Part model, mm, in its own coordinate system. Face numbers are marked on the shaded views. Give positions to 0.01 mm unless a question says otherwise; leave off trailing zeros. Loops run counter-clockwise (first coordinate to the right, second up) from the corner with the lowest first, then second, coordinate; pieces in that order, holes last. Notation, with made-up numbers: M -34.75,47 L -4.75,47 A20 ccw -4.75,86 Z; hole C 5,34.5 d5. An arc over 180 degrees is marked long. Answer in a Markdown table with one row per item.
from build123d import *

# Parameters (mm, degrees)
MAIN_BODY_DEPTH        = 53.8
SKETCH4_W              = 35
SKETCH4_H              = 10.428932188
SKETCH4_H_2            = 14.142135624
BOSS_EXTRUDE2_DEPTH    = 2
M2X0_4_TAPPED_HOLE2_D  = 1.6
SIDE_HOLES_D           = 2.9
FILLET1_R              = 0.5
BOSS_EXTRUDE4_START    = -10
BOSS_EXTRUDE4_DEPTH    = 10
M2_5_CLEARANCE_HOLE1_D = 2.9
M2_5_CLEARANCE_HOLE2_D = 2.9


# Read off the part's stored shape, not the designer's step: Boss-Extrude4
with BuildPart() as part:
    # Sketch1 → Main Body (new, symmetric)
    with BuildSketch(Plane.XY):
        Polygon((-7.5, 2.5), (2.5, 2.5), (2.5, -7.5), align=None)
    extrude(amount=MAIN_BODY_DEPTH, both=True)

    # Sketch4 → Boss-Extrude2 (add)
    with BuildSketch(Plane(origin=(-2.5, -2.5, 0), x_dir=(0, 0, 1), z_dir=(-0.7071067811865474, -0.7071067811865477, 0))):
        with Locations((0, 12.285533906)):
            Rectangle(SKETCH4_W, SKETCH4_H)
        Rectangle(SKETCH4_W, SKETCH4_H_2)
        with Locations((0, -12.285533906)):
            Rectangle(SKETCH4_W, SKETCH4_H)
        with BuildLine():
            Line((-17.5, -17.5), (-17.5, -7.071067812))
            Line((-17.5, -7.071067812), (-26.575364532, -7.071067812))
            ThreePointArc((-26.575364532, -7.071067812), (0, -27.5), (26.575364532, -7.071067812))
            Line((26.575364532, -7.071067812), (17.5, -7.071067812))
            Line((17.5, -7.071067812), (17.5, -17.5))
            Line((17.5, -17.5), (-17.5, -17.5))
        make_face()
        with BuildLine():
            Line((-17.5, -7.071067812), (-17.5, 7.071067812))
            Line((-17.5, 7.071067812), (-26.575364532, 7.071067812))
            ThreePointArc((-26.575364532, 7.071067812), (-27.5, 0), (-26.575364532, -7.071067812))
            Line((-26.575364532, -7.071067812), (-17.5, -7.071067812))
        make_face()
        with BuildLine():
            Line((-17.5, 7.071067812), (-17.5, 17.5))
            Line((-17.5, 17.5), (17.5, 17.5))
            Line((17.5, 17.5), (17.5, 7.071067812))
            Line((17.5, 7.071067812), (26.575364532, 7.071067812))
            ThreePointArc((26.575364532, 7.071067812), (0, 27.5), (-26.575364532, 7.071067812))
            Line((-26.575364532, 7.071067812), (-17.5, 7.071067812))
        make_face()
        with BuildLine():
            Line((26.575364532, 7.071067812), (17.5, 7.071067812))
            Line((17.5, 7.071067812), (17.5, -7.071067812))
            Line((17.5, -7.071067812), (26.575364532, -7.071067812))
            ThreePointArc((26.575364532, -7.071067812), (27.267861345, -3.565632859), (27.5, 0))
            ThreePointArc((27.5, 0), (27.267861345, 3.565632859), (26.575364532, 7.071067812))
        make_face()
    extrude(amount=-BOSS_EXTRUDE2_DEPTH)

    # M2x0.4 Tapped Hole2 (through all)
    with Locations(Plane(origin=(-2.5, -2.5, 0), x_dir=(-0.7071067811865477, 0.7071067811865474, 0), z_dir=(-0.7071067811865474, -0.7071067811865477, 0))):
        with Locations((-21, 0), (14, 21), (14, -21)):
            Hole(M2X0_4_TAPPED_HOLE2_D / 2)

    # Side holes (through all)
    with Locations(Plane.XY.offset(53.8)):
        with Locations((-1, -1)):
            Hole(SIDE_HOLES_D / 2)

    # Sketch8 → Revolve1 (revolve)
    with BuildSketch(Plane(origin=(0, 0, 0), x_dir=(0, 0, 1), z_dir=(0.7071067811865476, -0.7071067811865476, 0)), mode=Mode.PRIVATE) as revolve1_sk:
        with BuildLine():
            Line((0, 3.535533906), (0, 4.535533906))
            ThreePointArc((0, 4.535533906), (-4.596194078, 6.439339828), (-6.5, 11.035533906))
            Line((-6.5, 11.035533906), (-12, 3.535533906))
            Line((-12, 3.535533906), (0, 3.535533906))
        make_face()
    revolve(revolve1_sk.sketch.rotate(Axis((-2.5, -2.5, 0), (-0.7071067811865476, -0.7071067811865476, 0)), 270), axis=Axis((-2.5, -2.5, 0), (-0.7071067811865476, -0.7071067811865476, 0)))

    # Fillet1
    fillet1_edges = [part.edges().sort_by_distance(p)[0] for p in [
        (-3.207106781, -12.399494937, 0),
    ]]
    fillet(fillet1_edges, radius=FILLET1_R)

    # Boss-Extrude4 outline → Boss-Extrude4 (add)
    with BuildSketch(Plane(origin=(2.5, 0, 0), x_dir=(0, 0, -1), z_dir=(1, 0, 0)).offset(BOSS_EXTRUDE4_START)):
        Polygon((53.8, 33.99997125), (-53.8, 33.99997125), (-53.8, 23.99997125), (-14.986093738, 13.249985625), (-53.8, 2.5), (-23.827812525, 2.5), (0, 9.099403842), (23.827812525, 2.5), (53.8, 2.5), (14.986093738, 13.249985625), (53.8, 23.99997125), align=None)
        Polygon((23.827812525, 23.99997125), (0, 17.400567408), (-23.827812525, 23.99997125), align=None, mode=Mode.SUBTRACT)
    extrude(amount=BOSS_EXTRUDE4_DEPTH)

    # M2.5 Clearance Hole1 (through all)
    with Locations(Plane.XY.offset(53.8)):
        with Locations((-1, 28.99997125)):
            Hole(M2_5_CLEARANCE_HOLE1_D / 2)

    # M2.5 Clearance Hole2 (through all)
    with Locations(Plane(origin=(2.5, 0, 0), x_dir=(0, 0, -1), z_dir=(1, 0, 0))):
        with Locations((-43.8, -1.085786438), (43.8, -1.085786438)):
            Hole(M2_5_CLEARANCE_HOLE2_D / 2)


solid = part.part
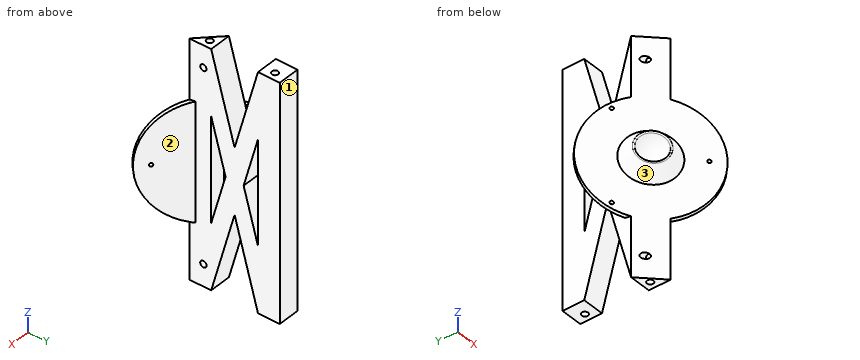
(1) Drill centre lines: line 1 along Y through (x, z) = (-0.5, -43.8); line 2 along Y through (x, z) = (-1.5, 43.8); line 3 along Y through (x, z) = (-5.5, 6.5). Where is each one in solid material? Low to high.
Recorded:
| item | result |
|---|---|
| line 1 | y = -4.5 to -2.54, 0.36 to 5.27, 21.23 to 27.64, 30.36 to 34 |
| line 2 | y = -3.5 to -2.54, 0.36 to 5.27, 21.23 to 27.64, 30.36 to 34 |
| line 3 | y = -8.9 to 3.33, 7.3 to 19.2, 24 to 34 |
(2) Saw through at A-A (z = -36). Write the cut outline in (x, y), plus the area to 3 significant figures.
Recorded:
| item | result |
|---|---|
| outline | M -7.5,2.5 L 2.5,-7.5 L 2.5,7.43 L -7.5,7.43 Z; M -7.5,19.07 L 2.5,19.07 L 2.5,34 L -7.5,34 Z; hole C -1,-1 d2.9; hole C -1,29 d2.9 |
| area | 235 mm^2 |
(3) Pin check, flat tips, straight feed: pin 1 Ø2 at (y, z) = (-4, -15) entering from -X; pin 2 Ø15.5 at (y, z) = (17.5, -23.5) entering from -X; pin 3 Ø4 at (y, z) = (1, -4) entering from -X; pin 4 Ø1.7 at (y, z) = (-1.09, 43.8) entering from +X. Stop position of each tip, or through.
Recorded:
| item | result |
|---|---|
| pin 1 | stops at x = -2 |
| pin 2 | stops at x = -17.41 |
| pin 3 | stops at x = -11.66 |
| pin 4 | passes through |
(4) Pull direction X, two halves, no side cores. Call the marked faces 1, 2 and 3: +X half, -X half, draft (parallel to the pull), parting line (faces both ways), or undercut.
Recorded:
| item | result |
|---|---|
| face 1 | draft |
| face 2 | +X half |
| face 3 | undercut |
